The model under review builds one solid part; all positions refer to its coordinate system, in mm. Round coordinates to 2 decimals unless told otherwise and drop trailing zeros. Write each loop counter-clockwise with the first axis right and the second up, starting at its lowest first coordinate (ties: lowest second). Pieces come first, ordered by that corner, then holes. Notation, with made-up numbers: (-15.5, -28.5) -> (-10.5, -28.5) arc R23 ccw to (-10.5, -13.5) -> close; hole circle Ø2 at (88, 89). An arc over 180 degrees is marked (long way). Return JSON: item names as keys, results as strings. Group by question number.
1. For line 1 along Y through (x, z) = (-67.9, 2.4); line 2 along Y through (x, z) = (-32, 2.6); line 3 along Y through (x, z) = (33, 0.25), list the stretches that pass through material, from the lowest coordinate up. Write a range as from..to.
2. Take a section at B-B, the plane x = -67.9. Write out the cut boundary in (y, z).
3. Mouldability with a two-part tool opening along X and no side actions: class faces 1 (the flat face through (-19, 47.1, 2)), 2 (the cylindrical face through (27.39, -27.78, 2.46)), 3 (the flat face through (-82.9, -19, 2)) as pulls with the +X half, pulls with the -X half, needs draft (parallel to the pull), parting line crosses it, or undercut.
4. Clearance check with flat-ended pins moving along their axes: P1, Ø13, axis at x = 0, y = 0, coming from the -Z side; P2, Ø14.5, axis at x = 32, y = -32, coming from the +Z side. State where each tip first meets the part, or that it passes through.
5. Take a section at C-C, the plane y = -32. Write out the cut boundary in (x, z), then the cut area to 3 significant figures.
6. Take a section at A-A, the plane z = 1.6. Give the number of separate pieces and of enclosed holes in the cut face, then the cut area to 3 significant figures.
from build123d import *

# Parameters (mm, degrees)
SKETCH_1_W      = 130
SKETCH_1_H      = 130
SKETCH_1_R      = 6.25
SKETCH_1_R_2    = 4
SKETCH_1_R_3    = 11
EXTRUDE_1_DEPTH = 5


with BuildPart() as part:
    # 草图1 → 凸台-拉伸1 (new body)
    with BuildSketch(Plane.XY):
        with Locations((-17.9, -17.9)):
            Rectangle(SKETCH_1_W, SKETCH_1_H)
        with Locations((-32, -32)):
            Circle(SKETCH_1_R, mode=Mode.SUBTRACT)
        with Locations((-32, 32)):
            Circle(SKETCH_1_R, mode=Mode.SUBTRACT)
        with Locations((32, 32)):
            Circle(SKETCH_1_R, mode=Mode.SUBTRACT)
        with Locations((32, -32)):
            Circle(SKETCH_1_R, mode=Mode.SUBTRACT)
        with Locations((-67.9, 32.1)):
            Circle(SKETCH_1_R_2, mode=Mode.SUBTRACT)
        with Locations((-67.9, -17.9)):
            Circle(SKETCH_1_R_2, mode=Mode.SUBTRACT)
        with Locations((-67.9, -67.9)):
            Circle(SKETCH_1_R_2, mode=Mode.SUBTRACT)
        with Locations((-17.9, -67.9)):
            Circle(SKETCH_1_R_2, mode=Mode.SUBTRACT)
        with Locations((32.1, -67.9)):
            Circle(SKETCH_1_R_2, mode=Mode.SUBTRACT)
        Circle(SKETCH_1_R_3, mode=Mode.SUBTRACT)
    extrude(amount=EXTRUDE_1_DEPTH)


solid = part.part
Output:
{
 "1": {"line 1": "y = -82.9..-71.9, -63.9..-21.9, -13.9..28.1, 36.1..47.1", "line 2": "y = -82.9..-38.25, -25.75..25.75, 38.25..47.1", "line 3": "y = -82.9..-71.8, -64..-38.17, -25.83..25.83, 38.17..47.1"},
 "2": {"outline": "(-82.9, 0) -> (-71.9, 0) -> (-71.9, 5) -> (-82.9, 5) -> close; (-63.9, 0) -> (-21.9, 0) -> (-21.9, 5) -> (-63.9, 5) -> close; (-13.9, 0) -> (28.1, 0) -> (28.1, 5) -> (-13.9, 5) -> close; (36.1, 0) -> (47.1, 0) -> (47.1, 5) -> (36.1, 5) -> close"},
 "3": {"face 1": "needs draft", "face 2": "undercut", "face 3": "pulls with the -X half"},
 "4": {"P1": "passes through", "P2": "stops at z = 5"},
 "5": {"outline": "(-82.9, 0) -> (-38.25, 0) -> (-38.25, 5) -> (-82.9, 5) -> close; (-25.75, 0) -> (25.75, 0) -> (25.75, 5) -> (-25.75, 5) -> close; (38.25, 0) -> (47.1, 0) -> (47.1, 5) -> (38.25, 5) -> close", "area": "525 mm^2"},
 "6": {"separate pieces": "1", "enclosed holes": "10", "area": "15,800 mm^2"}
}
